The listing builds one solid part. Answer for the finished solid, in the listing's coordinates (mm). Face numbers are marked on the shaded views. A direction names the side the tool comes from. Coordinates: 2 decimals unless noted, no trailing zeros. Order: outer loops, then holes, each group sorted by start corner. A loop starts at its lowest first (then second) coordinate and runs counter-clockwise, first axis right, second up. Notation, with made-up numbers: (-34.75, 0) - (11.25, 0) arc R15 ccw to (11.25, 6) - close; hole circle Ø5 at (7, 29). An arc over 180 degrees is marked (long way). One line per item, written item: value. Start each with the question number.
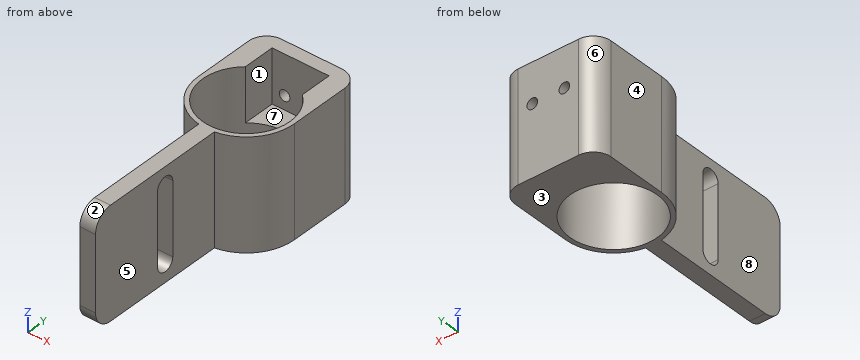
```python
from build123d import *

# Parameters (mm, degrees)
SKETCH1_R           = 12.25
BOSS_EXTRUDE2_DEPTH = 31
SKETCH2_W           = 16
SKETCH2_H           = 9
CUT_EXTRUDE1_DEPTH  = 15
SKETCH3_R           = 1.5
CUT_EXTRUDE2_DEPTH  = 15
CUT_EXTRUDE3_DEPTH  = 15
FILLET1_R           = 5


with BuildPart() as part:
    # Sketch1 → Boss-Extrude2 (new body)
    with BuildSketch(Plane.XY):
        with BuildLine():
            Line((-13.5, 0), (-13.5, 22))
            Line((-13.5, 22), (13.5, 22))
            Line((13.5, 22), (13.5, 0))
            ThreePointArc((13.5, 0), (10.279789156, -8.750767675), (2.155417052, -13.326821727))
            Line((2.155417052, -13.326821727), (2.155417052, -53.326821727))
            Line((2.155417052, -53.326821727), (-2.26470283, -53.326821727))
            Line((-2.26470283, -53.326821727), (-2.26470283, -13.308685927))
            ThreePointArc((-2.26470283, -13.308685927), (-10.315606822, -8.708516286), (-13.5, 0))
        make_face()
        Circle(SKETCH1_R, mode=Mode.SUBTRACT)
    extrude(amount=BOSS_EXTRUDE2_DEPTH)

    # Sketch2 → Cut-Extrude1 (cut)
    with BuildSketch(Plane.XY.offset(31)):
        with Locations((0, 13.776987658)):
            Rectangle(SKETCH2_W, SKETCH2_H)
    extrude(amount=-CUT_EXTRUDE1_DEPTH, mode=Mode.SUBTRACT)

    # Sketch3 → Cut-Extrude2 (cut)
    with BuildSketch(Plane.XZ.offset(-18.276987658)):
        with Locations(Location((-4.5, 19.859972316, 0), (0, 0, 270))):
            Circle(SKETCH3_R)
        with Locations(Location((4.5, 19.859972316, 0), (0, 0, 270))):
            Circle(SKETCH3_R)
    extrude(amount=-CUT_EXTRUDE2_DEPTH, mode=Mode.SUBTRACT)

    # Sketch4 → Cut-Extrude3 (cut)
    with BuildSketch(Plane(origin=(2.155417052, 0, 0), x_dir=(0, 0, -1), z_dir=(1, 0, 0))):
        with BuildLine():
            Line((-25.787321286, -27.326821727), (-5.462583223, -27.326821727))
            ThreePointArc((-5.462583223, -27.326821727), (-2.912583223, -29.876821727), (-5.462583223, -32.426821727))
            Line((-5.462583223, -32.426821727), (-25.787321286, -32.426821727))
            ThreePointArc((-25.787321286, -32.426821727), (-28.337321286, -29.876821727), (-25.787321286, -27.326821727))
        make_face()
    extrude(amount=-CUT_EXTRUDE3_DEPTH, mode=Mode.SUBTRACT)

    # Fillet1
    fillet1_edges = [part.edges().sort_by_distance(p)[0] for p in [
        (-0.054642889, -53.326821727, 0),
        (-0.054642889, -53.326821727, 31),
        (-13.5, 22, 15.5),
        (13.5, 22, 15.5),
    ]]
    fillet(fillet1_edges, radius=FILLET1_R)


solid = part.part
```
(1) The part is cut by section A-A on z = 7. Determine the outline of the cut face in (x, y), plus the area to 3 significant figures.
(2) For a pull along Y with two mould halves and no side action, classify the marked faces 1, 2 and 3 as pulls with the +Y half, pulls with the -Y half, needs draft (parallel to the pull), parting line crosses it, or undercut.
(3) Flat-ended cylindrical pins translate along their axes: pin 1 Ø2.5 at (x, z) = (4.5, 19.86) entering from +Y; pin 2 Ø10 at (y, z) = (-17, 18.5) entering from +X; pin 3 Ø3 at (x, z) = (-10.5, 22.5) entering from -Y. Find the tip coordinate at first contact, or state that the pin passes through.
(4) Consider probe 1 along Y at (x, z) = (0, 11.5); probe 2 along X at (y, z) = (-0.5, 22); probe 3 along X at (y, z) = (11.5, 23). Determine where each line is inside the solid, lowest interval first.
(5) The part is cut by section D-D on z = 29.5. Determine the outline of the cut face in (x, y), plus the area to 3 significant figures.
(6) The part is cut by section B-B on x = 0. Determine the outline of the cut face in (y, z), plus the area to 3 significant figures.
(7) The part is cut by section C-C on x = -10.75. Determine the outline of the cut face in (y, z).
(8) For the marked faces 4, 5, 6, 7 and 8, determine the directions among +Z, -Z, +X, -X, +Y, -Y from which every point of the face is accessible in a straight line to the end or side of a thin tool.
Completed:
1. outline: (-13.5, 0) arc R13.5 ccw to (-2.26, -13.31) - (-2.26, -27.33) - (2.16, -27.33) - (2.16, -13.33) arc R13.5 ccw to (13.5, 0) - (13.5, 17) arc R5 ccw to (8.5, 22) - (-8.5, 22) arc R5 ccw to (-13.5, 17) - close; (-2.26, -53.33) - (2.16, -53.33) - (2.16, -32.43) - (-2.26, -32.43) - close; hole circle Ø24.5 at (0, 0)
1. area: 552 mm2
2. face 1: undercut
2. face 2: pulls with the -Y half
2. face 3: needs draft
3. pin 1: stops at y = -10.82
3. pin 2: stops at x = 6.18
3. pin 3: stops at y = -10.06
4. probe 1: y = -53.33 to -32.43, -27.33 to -12.25, 12.25 to 22
4. probe 2: x = -13.49 to -12.24, 12.24 to 13.49
4. probe 3: x = -13.5 to -8, 8 to 13.5
5. outline: (-13.5, 0) arc R13.5 ccw to (-2.26, -13.31) - (-2.26, -51.9) - (2.16, -51.9) - (2.16, -13.33) arc R13.5 ccw to (13.5, 0) - (13.5, 17) arc R5 ccw to (8.5, 22) - (-8.5, 22) arc R5 ccw to (-13.5, 17) - close; hole (-8, 9.28) arc R12.25 ccw (long way) to (8, 9.28) - (8, 18.28) - (-8, 18.28) - close
5. area: 457 mm2
6. outline: (-53.33, 5) arc R5 ccw to (-48.33, 0) - (-12.25, 0) - (-12.25, 31) - (-48.33, 31) arc R5 ccw to (-53.33, 26) - close; (12.25, 0) - (22, 0) - (22, 31) - (18.28, 31) - (18.28, 16) - (12.25, 16) - close; hole (-32.43, 5.46) arc R2.55 ccw to (-27.33, 5.46) - (-27.33, 25.79) arc R2.55 ccw to (-32.43, 25.79) - close
6. area: 1,350 mm2
7. outline: (-8.17, 0) - (-5.87, 0) - (-5.87, 31) - (-8.17, 31) - close; (5.87, 0) - (21.47, 0) - (21.47, 31) - (5.87, 31) - close
8. face 4: +Z, -Z, -X, +Y, -Y
8. face 5: +Z, -Z, +X, -Y
8. face 6: +Z, -Z, -X, +Y
8. face 7: +Z
8. face 8: +Z, -Z, -X, -Y
